Geometry: final body of the model. Coordinates: model frame, mm. A direction names the side the tool comes from. Coordinates: 2 decimals unless noted, no trailing zeros. Write each loop counter-clockwise with the first axis right and the second up, starting at its lowest first coordinate (ties: lowest second). Pieces come first, ordered by that corner, then holes. Notation, with made-up numbers: M 82.25,54 L 117.25,54 A21 cw 117.25,78 Z; hole C -31.75,-19.75 d2. An arc over 180 degrees is marked long. Write item = value, one per line. Start each with the question number.
Item 1: Section D-D on x = 16.5. Output: boundary loops of the cut face in (y, z), plus the area to 3 significant figures.
Item 2: First-contact query: pin 1 Ø5 at (x, z) = (0, 18.21) entering from +Y (3 decimals); pin 2 Ø12 at (x, z) = (-2.5, 13) entering from +Y; pin 3 Ø8 at (x, y) = (7, -14.5) entering from -Z; pin 4 Ø1.6 at (x, z) = (-35.5, 28) entering from +Y. Flat tips, straight axial feed; report the tip coordinate or a pass-through.
Item 3: Ray query, L1, parallel to X at y = -13.75, z = 15.5; L2, parallel to Z at x = 0, y = -29.1; L3, parallel to Z at x = 21, y = -20.25. Return the intervals inside material, ascending. Write a range as [from, to].
Item 4: Section C-C on z = 19. Output: boundary loops of the cut face in (x, y).
Item 5: Section B-B on x = 0. Output: boundary loops of the cut face in (y, z), plus the area to 3 significant figures.
Item 6: Reachability of faces 4 (the cylindrical face through (-0.65, -28.52, 15.28)), 5 (the flat face through (-34.841, -13, 15)), 6 (the flat face through (-36, -10, 28)), 7 (the cylindrical face through (36.55, -0.43, 13.69)) from +Z, -Z, +X, -X, +Y, -Y: full face, straight path, thin tool, end or side. Return the list, or none.
Item 7: Pull-direction query (Z, two-part tool) for faces 1 (the cylindrical face through (-36.55, -0.43, 13.31)), 2 (the flat face through (0, -28, 0)), 3 (the flat face through (36, -5, 27)); classes: +Z half, -Z half, draft (parallel to the pull), parting line (faces both ways), or undercut.
Item 8: Section A-A on y = -2.5. Output: boundary loops of the cut face in (x, z), plus the area to 3 significant figures.
from build123d import *

# Parameters (mm, degrees)
F2_DEPTH = 30
F3_DEPTH = 27
F4_W     = 10
F4_H     = 2
F5_DEPTH = 74.5
F6_R     = 3
F7_DEPTH = 25
F8_R     = 1.5


with BuildPart() as f2:
    # F0 (on Front) → F2 (new body)
    with BuildSketch(Plane.XZ):
        Polygon((-37, 0), (0, 0), (37, 0), (37, 32), (-37, 32), align=None)
    extrude(amount=F2_DEPTH)

    # F1 (on face) → F3 (cut)
    with BuildSketch(Plane.XZ):
        Polygon((-34.841463, 29), (-34.841463, 0), (0, 0), (35.158537, 0), (35.158537, 29), align=None)
    extrude(amount=F3_DEPTH, mode=Mode.SUBTRACT)

    # F4 (on face) → F5 (cut)
    with BuildSketch(Plane(origin=(-37, 0, 0), x_dir=(0, -1, 0), z_dir=(-1, 0, 0))):
        with Locations((5, 28)):
            Rectangle(F4_W, F4_H)
    extrude(amount=-F5_DEPTH, mode=Mode.SUBTRACT)

    # F6 (on face) → F7 (cut)
    with BuildSketch(Plane.XZ.offset(30)):
        with Locations((0, 18.206734)):
            Circle(F6_R)
    extrude(amount=-F7_DEPTH, mode=Mode.SUBTRACT)

    # F8
    f8_edges = [f2.edges().sort_by_distance(p)[0] for p in [
        (37, -15, 0),
        (0, 0, 32),
        (-37, -15, 0),
        (-37, 0, 13.5),
        (37, 0, 13.5),
    ]]
    fillet(f8_edges, radius=F8_R)


solid = f2.part
Responses:
q1.outline = M -30,0 L -27,0 L -27,29 L 0,29 L 0,30.5 A1.5 ccw -1.5,32 L -30,32 Z
q1.area = 177 mm²
q2.pin_1 = through
q2.pin_2 = -27
q2.pin_3 = 29
q2.pin_4 = -10
q3.L1 = [-37, -34.84], [35.16, 37]
q3.L2 = [0, 15.21], [21.21, 32]
q3.L3 = [29, 32]
q4.outline = M -37,-30 L -2.89,-30 L -2.89,-27 L -34.84,-27 L -34.84,0 L -35.5,0 A1.5 ccw -37,-1.5 Z; M 2.89,-30 L 37,-30 L 37,-1.5 A1.5 ccw 35.5,0 L 35.16,0 L 35.16,-27 L 2.89,-27 Z
q5.outline = M -30,0 L -27,0 L -27,15.21 L -30,15.21 Z; M -30,21.21 L -27,21.21 L -27,29 L 0,29 L 0,30.5 A1.5 ccw -1.5,32 L -30,32 Z
q5.area = 159 mm²
q6.face_4 = +Y, -Y
q6.face_5 = -Z, +Y
q6.face_6 = +X, -X, +Y
q6.face_7 = -Z, +X, +Y
q7.face_1 = draft
q7.face_2 = -Z half
q7.face_3 = undercut
q8.outline = M -37,1.5 A1.5 ccw -35.5,0 L -34.84,0 L -34.84,27 L -37,27 Z; M -37,29 L 37,29 L 37,32 L -37,32 Z; M 35.16,0 L 35.5,0 A1.5 ccw 37,1.5 L 37,27 L 35.16,27 Z
q8.area = 329 mm²
